```python
from build123d import *

# Parameters (mm, degrees)
SKETCH1_R           = 1.5
BOSS_EXTRUDE1_DEPTH = 3
CUT_EXTRUDE2_DEPTH  = 0.9
SKETCH5_W           = 3.6
SKETCH5_H           = 3
FILLET1_R           = 2.5


with BuildPart() as part:
    # Sketch1 → Boss-Extrude1 (new body)
    with BuildSketch(Plane.XY.offset(1.9)):
        with BuildLine():
            Line((2.5, 8.124038405), (2.5, 41))
            ThreePointArc((2.5, 41), (0, 43.5), (-2.5, 41))
            Line((-2.5, 41), (-2.5, 8.124038405))
            ThreePointArc((-2.5, 8.124038405), (-2.735010245, 8.047963653), (-2.967710696, 7.965092167))
            Line((-2.967710696, 7.965092167), (-3.054167872, 8.093270203))
            ThreePointArc((-3.054167872, 8.093270203), (-4.342095244, 9.472160372), (-5.994566265, 10.382893341))
            ThreePointArc((-5.994566265, 10.382893341), (-6.032083889, 8.496444973), (-5.481893659, 6.691622066))
            Line((-5.481893659, 6.691622066), (-5.414116812, 6.552658937))
            ThreePointArc((-5.414116812, 6.552658937), (-6.01040764, 6.01040764), (-6.552658937, 5.414116812))
            Line((-6.552658937, 5.414116812), (-6.691622066, 5.481893659))
            ThreePointArc((-6.691622066, 5.481893659), (-8.496444973, 6.032083889), (-10.382893341, 5.994566265))
            ThreePointArc((-10.382893341, 5.994566265), (-9.472160372, 4.342095244), (-8.093270203, 3.054167872))
            Line((-8.093270203, 3.054167872), (-7.965092167, 2.967710696))
            ThreePointArc((-7.965092167, 2.967710696), (-8.210369523, 2.199961883), (-8.381827508, 1.41243323))
            Line((-8.381827508, 1.41243323), (-8.536061531, 1.401648136))
            ThreePointArc((-8.536061531, 1.401648136), (-10.374179133, 0.975715399), (-11.989132531, 0))
            ThreePointArc((-11.989132531, 0), (-10.374179133, -0.975715399), (-8.536061531, -1.401648136))
            Line((-8.536061531, -1.401648136), (-8.381827508, -1.41243323))
            ThreePointArc((-8.381827508, -1.41243323), (-8.210369523, -2.199961883), (-7.965092167, -2.967710696))
            Line((-7.965092167, -2.967710696), (-8.093270203, -3.054167872))
            ThreePointArc((-8.093270203, -3.054167872), (-9.472160372, -4.342095244), (-10.382893341, -5.994566265))
            ThreePointArc((-10.382893341, -5.994566265), (-8.496444973, -6.032083889), (-6.691622066, -5.481893659))
            Line((-6.691622066, -5.481893659), (-6.552658937, -5.414116812))
            ThreePointArc((-6.552658937, -5.414116812), (-6.01040764, -6.01040764), (-5.414116812, -6.552658937))
            Line((-5.414116812, -6.552658937), (-5.481893659, -6.691622066))
            ThreePointArc((-5.481893659, -6.691622066), (-6.032083889, -8.496444973), (-5.994566265, -10.382893341))
            ThreePointArc((-5.994566265, -10.382893341), (-4.342095244, -9.472160372), (-3.054167872, -8.093270203))
            Line((-3.054167872, -8.093270203), (-2.967710696, -7.965092167))
            ThreePointArc((-2.967710696, -7.965092167), (-2.200030635, -8.210351101), (-1.412573605, -8.381803852))
            Line((-1.412573605, -8.381803852), (-1.393124693, -8.60968341))
            ThreePointArc((-1.393124693, -8.60968341), (-0.957124189, -10.404769076), (-0.000200717, -11.984872381))
            ThreePointArc((-0.000200717, -11.984872381), (0.95677568, -10.404801129), (1.39283631, -8.609730068))
            Line((1.39283631, -8.609730068), (1.412292855, -8.381851161))
            ThreePointArc((1.412292855, -8.381851161), (2.199774454, -8.210495053), (2.967443903, -7.965191566))
            Line((2.967443903, -7.965191566), (3.392820223, -8.498315042))
            ThreePointArc((3.392820223, -8.498315042), (4.564279824, -9.615969997), (5.992088536, -10.379404655))
            ThreePointArc((5.992088536, -10.379404655), (6.04494749, -8.761172247), (5.662865105, -7.187805396))
            Line((5.662865105, -7.187805396), (5.413897328, -6.552840279))
            ThreePointArc((5.413897328, -6.552840279), (7.689867596, -3.621593069), (8.5, 0))
            ThreePointArc((8.5, 0), (6.837397166, 5.049752469), (2.5, 8.124038405))
        make_face()
        with Locations((0, 41)):
            Circle(SKETCH1_R, mode=Mode.SUBTRACT)
    extrude(amount=-BOSS_EXTRUDE1_DEPTH)

    # Sketch4 → Cut-Extrude2 (cut)
    with BuildSketch(Plane.XY.offset(1.9)):
        with BuildLine():
            Line((-5.102940329, -2.6), (-1.358771093, -3.333727811))
            ThreePointArc((-1.358771093, -3.333727811), (-3.6, 0), (-1.358771093, 3.333727811))
            Line((-1.358771093, 3.333727811), (-5.102940329, 2.6))
            Line((-5.102940329, 2.6), (-5.102940329, -2.6))
        make_face()
    extrude(amount=-CUT_EXTRUDE2_DEPTH, mode=Mode.SUBTRACT)

    # Sketch5 → Cut-Revolve1 (revolve, cut)
    with BuildSketch(Plane(origin=(0, 0, 0), x_dir=(1, 0, 0), z_dir=(0, 1, 0))):
        with Locations((1.8, -1.5)):
            Rectangle(SKETCH5_W, SKETCH5_H)
    revolve(axis=Axis((0, 0, 0), (0, 0, 1)), mode=Mode.SUBTRACT)

    # Chamfer1
    # the kernel refuses this chamfer: 1.996823512, 1.978396736, 1.94931332, 1.412365401 mm, written as the material it takes off along each edge
    with BuildSketch(Plane(origin=(5.992088536, -10.379404655, 6.233820359), x_dir=(-0.8794300447910056, 0.4760281465616188, 0), z_dir=(0, 0, -1))) as chamfer1_piece_1:
        with BuildLine():
            Line((1.679904515, 0), (0.570181749, 1.211368913))
            ThreePointArc((0.570181749, 1.211368913), (0.257488937, 0.635031779), (0, 0))
            ThreePointArc((0, 0), (0.866421107, -0.059071898), (1.679904515, 0))
        make_face()
    extrude(amount=11.667640718, mode=Mode.SUBTRACT)
    with BuildSketch(Plane(origin=(-0.000200717, -11.984872381, 6.284042251), x_dir=(0.553758056262258, 0.8326776177637093, 0), z_dir=(0, 0, -1))) as chamfer1_piece_2:
        with BuildLine():
            Line((1.33943628, 0), (0.703391742, -1.546031937))
            ThreePointArc((0.703391742, -1.546031937), (0.308543545, -0.822544611), (0, 0))
            ThreePointArc((0, 0), (0.684773692, 0.037130534), (1.33943628, 0))
        make_face()
    extrude(amount=11.768084503, mode=Mode.SUBTRACT)
    with BuildSketch(Plane(origin=(-5.994566265, -10.382893341, 6.307600342), x_dir=(0.8971018613244867, 0.44182377754953556, 0), z_dir=(0, 0, -1)), Plane(origin=(-10.382893341, -5.994566265, 6.307600342), x_dir=(0.9978248904640774, -0.06592031530834563, 0), z_dir=(0, 0, -1)), Plane(origin=(-11.989132531, 0, 6.307600342), x_dir=(0.8311815460161414, -0.5560011129145489, 0), z_dir=(0, 0, -1))) as chamfer1_piece_3:
        with BuildLine():
            Line((1.33889649, 0), (0.700148491, -1.556942978))
            ThreePointArc((0.700148491, -1.556942978), (0.305807457, -0.828670891), (0, 0))
            ThreePointArc((0, 0), (0.684607685, 0.037444556), (1.33889649, 0))
        make_face()
    extrude(amount=11.815200684, mode=Mode.SUBTRACT)
    with BuildSketch(Plane(origin=(-10.382893341, 5.994566265, 6.307600342), x_dir=(0.9993864811320993, 0.035023725250178994, 0), z_dir=(0, 0, -1)), Plane(origin=(-5.994566265, 10.382893341, 6.307600342), x_dir=(0.8830059434842266, -0.4693618047642254, 0), z_dir=(0, 0, -1))) as chamfer1_piece_4:
        with BuildLine():
            Line((1.707126049, 0), (0.549125448, 1.221108125))
            ThreePointArc((0.549125448, 1.221108125), (0.246629708, 0.639737105), (0, 0))
            ThreePointArc((0, 0), (0.881190909, -0.060960877), (1.707126049, 0))
        make_face()
    extrude(amount=11.815200684, mode=Mode.SUBTRACT)

    # Fillet1
    fillet1_edges = [part.edges().sort_by_distance(p)[0] for p in [
        (5.413897328, -6.552840279, 0.4),
    ]]
    fillet(fillet1_edges, radius=FILLET1_R)


solid = part.part
```
For this review, take the finished solid that the model builds, in its own axes (mm). A direction names the side the tool comes from. Coordinates: 2 decimals unless noted, no trailing zeros. Loops run counter-clockwise (first coordinate to the right, second up) from the corner with the lowest first, then second, coordinate; pieces in that order, holes last.
1. Add section B-B, the plane y = 23. Give the boundary of the cut face in (x, z), then the cut area to 3 significant figures.
2. Mouldability with a two-part tool opening along Y and no side actions: class faces 1 (the flat face through (-5.103, 0, 1.5)), 2 (the flat face through (-9.31, -5.3, 0.42)), 3 (the flat face through (-10.71, 0.07, 0.42)) as +Y half, -Y half, draft (parallel to the pull), parting line (faces both ways), or undercut.
3. Add section A-A, the plane x = 0. Give the boundary of the cut face in (y, z), then the cut area to 3 significant figures.
4. For line 1 (Y direction, x = -8.75, z = 1.6); line 2 (Y direction, x = 0, z = 1.3); line 3 (Y direction, x = -2.75, z = 0.1), list the stretches that pass through material, from the lowest coordinate up.
5. Insertion check: P1, Ø6, axis at x = 6, y = 17.5, coming from the -Z side; P2, Ø1.5, axis at x = 6, z = 1.5, coming from the +Y side; P3, Ø3, axis at x = -2.5, y = -1.5, coming from the +Z side; P4, Ø1.5, axis at y = 23.5, z = 1, coming from the +X side. Each pin has a flat end and moves straight along its axis. Give the tip position at first contact, or say it passes through.
6. For faces 4 (the cylindrical face through (-1.23, -9.58, 0.42)), 5 (the cylindrical face through (6.005, -8.452, 0.421)), 6 (the cylindrical face through (-5.91, 7.86, 0.42)), 7 (the cylindrical face through (-7.65, 5.85, 0.42)), 8 (the flat face through (-3.205, 2.972, 1.456)), list the 3-axis set-ups (+Z, -Z, +X, -X, +Y, -Y) from which the entire face can be reached by the end or side of a thin tool; tool diameter is ignored.
Result:
1. outline: (-2.5, -1.1) - (2.5, -1.1) - (2.5, 1.9) - (-2.5, 1.9) - close
1. area: 15.0 mm2
2. face 1: undercut
2. face 2: -Y half
2. face 3: +Y half
3. outline: (-10.72, -1.1) - (39.5, -1.1) - (39.5, 1.9) - (3.6, 1.9) - (3.6, 0) - (-3.6, 0) - (-3.6, 1.9) - (-10.72, 1.9) - close; (42.5, -1.1) - (43.5, -1.1) - (43.5, 1.9) - (42.5, 1.9) - close
3. area: 140 mm2
4. line 1: y = -6.06 to -3.57, -1.38 to 1.38, 3.57 to 5.97
4. line 2: y = -10.72 to -3.6, 3.6 to 39.5, 42.5 to 43.5
4. line 3: y = -8.04 to -2.32, 2.32 to 8.04
5. P1: passes through
5. P2: stops at y = 6.68
5. P3: stops at z = 1
5. P4: stops at x = 2.5
6. face 4: +Z, -Z, -Y
6. face 5: +Z, -Z, +X
6. face 6: +Z, -Z, -X
6. face 7: +Z, -Z, +Y
6. face 8: +Z
